Design review of the part built by this model. Coordinates are the model's own, in mm. A direction names the side the tool comes from. Give positions to 0.01 mm unless a question says otherwise; leave off trailing zeros. Loops run counter-clockwise (first coordinate to the right, second up) from the corner with the lowest first, then second, coordinate; pieces in that order, holes last. Notation, with made-up numbers: M 43,75 L 98,75 A23 ccw 98,91 Z; hole C 26.25,66 d3. An arc over 180 degrees is marked long. Use CSV: the item, a comma, the result in double quotes.
Autodesk Inventor part; units mm, degrees
ref_plane "YZ Plane" through (0, 0, 0) normal (1, 0, 0) x (0, 1, 0)
ref_plane "XZ Plane" through (0, 0, 0) normal (0, 1, 0) x (-1, 0, 0)
ref_plane "XY Plane" through (0, 0, 0) normal (0, 0, 1) x (1, 0, 0)
sketch "Sketch1" plane through (0, 0, 0) normal (0, 1, 0) x (-1, 0, 0)
  line L0 (-38.227, 25.527) -> (38.227, 25.527)
  line L1 (38.227, 25.527) -> (38.227, -25.527)
  line L2 (38.227, -25.527) -> (-38.227, -25.527)
  line L3 (-38.227, -25.527) -> (-38.227, 25.527)
  line L4 (-38.227, 25.527) -> (38.227, -25.527) construction
  point P0 (0, 0)
  point P1 (0, 0)
  dimension "d0" = 76.454
  dimension "d1" = 51.054
extrude "Extrusion1" add sketch "Sketch1" along normal blind 1.524
sketch "Sketch2" plane through (0, 1.524, 0) normal (0, 1, 0) x (1, 0, 0)
  line L0 (-38.227, -25.527) -> (38.227, -25.527)
  line L1 (38.227, -25.527) -> (38.227, 25.527)
  line L2 (38.227, 25.527) -> (-38.227, 25.527)
  line L3 (-38.227, 25.527) -> (-38.227, -25.527)
  circle A0 centre (-35.179, 22.479) radius 1.524
  circle A1 centre (-35.179, -22.479) radius 1.524
  circle A2 centre (35.179, 22.479) radius 1.524
  circle A3 centre (35.179, -22.479) radius 1.524
  point P0 (0, 0)
  dimension "d4" = 3.048
  dimension "d5" = 3.048
  dimension "d6" = 3.048
  dimension "d7" = 3.048
  dimension "d8" = 3.048
  dimension "d9" = 3.048
  dimension "d10" = 3.048
  dimension "d11" = 3.048
  dimension "d12" = 3.048
extrude "Extrusion2" cut sketch "Sketch2" against normal up to next contours A0 | A1 | A2 | A3
sketch "Sketch6" plane through (0, 1.524, 0) normal (0, 1, 0) x (1, 0, 0)
  line L0 (38.227, -25.527) -> (-0.127, -25.527)
  line L1 (-0.127, -25.527) -> (-0.127, 13.335)
  line L2 (-0.127, 13.335) -> (38.227, 13.335)
  line L3 (38.227, 13.335) -> (38.227, -25.527)
  line L4 (23.495, 18.415) -> (24.003, 18.415)
  line L5 (38.227, 25.527) -> (-38.227, 25.527)
  line L6 (-38.227, 25.527) -> (-38.227, -25.527)
  point P0 (0, 0)
  dimension "d23" = 12.192
  dimension "d24" = 38.1
extrude "Extrusion3" cut sketch "Sketch6" against normal blind 25.4
properties part number "MainBoard" material "Silicon Nitride"
(1) We need section A-A on y = 0.6. State the section outline as (x, z) points (3 decimals).
A:
outline,"M -38.227,-25.527 L 38.227,-25.527 L 38.227,-13.335 L -0.127,-13.335 L -0.127,25.527 L -38.227,25.527 Z; hole C -35.179,-22.479 d3.048; hole C -35.179,22.479 d3.048; hole C 35.179,-22.479 d3.048"
(2) Machinability: for faces 4 (the flat face through (-0.127, 1, 6)), 5 (the flat face through (38.227, 1, -20)), which of the approach directions +Z, -Z, +X, -X, +Y, -Y give a long, thin tool a straight path to every point of the face, cutting with its end or side? Answer none if there is none.
A:
face 4,"+Z, +X, +Y, -Y"
face 5,"+Z, -Z, +X, +Y, -Y"
(3) We need section B-B on z = -10.5. State the section outline as (x, y) points, then the cut area to 3 significant figures.
A:
outline,"M -38.23,0 L -0.13,0 L -0.13,1.52 L -38.23,1.52 Z"
area,"58.1 mm²"
(4) Wall thickness on line 1 along X through (y, z) = (1.3, -23); line 2 along X through (y, z) = (0.1, 22.5); line 3 along X through (y, z) = (1.45, -8): over which ranges is each line inside the solid? List them lowest first. Write a range as [from, to].
A:
line 1,"[-38.23, -36.61], [-33.75, 33.75], [36.61, 38.23]"
line 2,"[-38.23, -36.7], [-33.66, -0.13]"
line 3,"[-38.23, -0.13]"
(5) The part is to be moulded in two halves that separate along X. For faces 1 (the flat face through (-16, 0, -5)), 2 (the cylindrical face through (36.59, 0.77, -21.9)), 3 (the flat face through (-38.227, 1, 0)), say which applies: released by +X, released by -X, zero draft, split by the parting line, or undercut.
A:
face 1,"zero draft"
face 2,"undercut"
face 3,"released by -X"
(6) Clearance check with a flat-ended pin moving along its axis: P1, Ø10, axis at x = 5, z = 2.5, coming from the -Y side. State where the tip first meets the part, or that it passes through.
A:
P1,"through"
(7) We need section C-C on x = 13. State the section outline as (y, z) points (3 decimals).
A:
outline,"M 0,-25.527 L 1.524,-25.527 L 1.524,-13.335 L 0,-13.335 Z"
